CAD build for the part. Positions are in the model's coordinates, mm. Face numbers are marked on the shaded views. A direction names the side the tool comes from. Give positions to 0.01 mm unless a question says otherwise; leave off trailing zeros. Order: outer loops, then holes, each group sorted by start corner. A loop starts at its lowest first (then second) coordinate and runs counter-clockwise, first axis right, second up.
Item 1: Flat gauge pins, fed straight in: P1, Ø9.5, axis at y = 8, z = 0.5, coming from the -X side; P2, Ø7, axis at x = -80, z = -13, coming from the +Y side. Where does each tip first touch, or does it go through?
Item 2: Band-saw the part on C-C on x = -37.5. Give the cut face in (y, z).
Item 3: Which spindle directions (+Z, -Z, +X, -X, +Y, -Y) get a long thin tool onto all of the face, cutting with end or side? Do the marked faces 1, 2 and 3. Say none if no direction does.
Item 4: Band-saw the part on D-D on y = 3.75. Count the separate pieces of the cut face and the enclosed holes in it, plus the area to 3 significant figures.
Item 5: Band-saw the part on B-B on x = -80. Give the cut face in (y, z), plus the area to 3 significant figures.
Item 6: Two-plate mould, pull along X, no slides. Class the marked faces 4, 5, 6 and 7: released by +X, released by -X, zero draft, split by the parting line, or undercut.
Item 7: Band-saw the part on A-A on x = -11.25. Give the cut face in (y, z), plus the area to 3 significant figures.
Item 8: Wall check: L1, parallel to Z at x = -80, y = 6; L2, parallel to Z at x = -74.5, y = 5; L3, parallel to X at y = 8.5, z = 1. Give the ranges that are in metal, low to high.
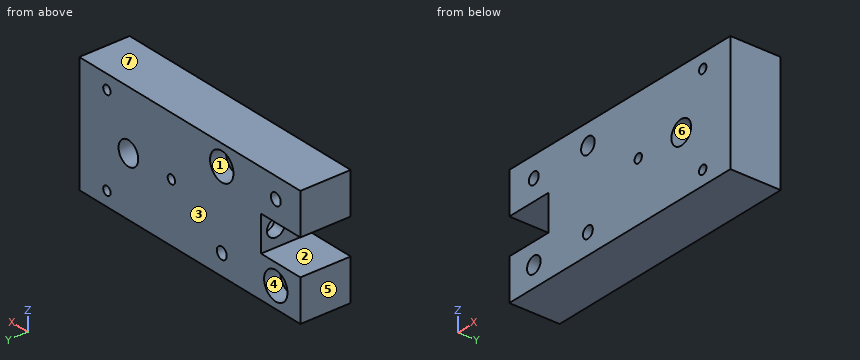
```python
from build123d import *

# Parameters (mm, degrees)
EXTRUDE_1_DEPTH        = 17
SKETCH_4_R             = 2.75
SKETCH_4_R_2           = 2
SKETCH_4_R_3           = 4
SKETCH_4_R_4           = 1.5
CUT_EXTRUDE_2_DEPTH    = 18
SKETCH_5_R             = 4.75
CUT_EXTRUDE_3_DEPTH    = 5.4
HOLE_WIZARD_M4_1_D     = 6
HOLE_WIZARD_M4_1_DEPTH = 4
HOLE_WIZARD_M4_1_TIP   = 1.802581857


with BuildPart() as part:
    # 스케치1 → 보스-돌출1 (new body)
    with BuildSketch(Plane(origin=(0, 0, 0), x_dir=(1, 0, 0), z_dir=(0, 1, 0))):
        Polygon((-90, -6), (-90, -20), (0, -20), (0, 20), (-90, 20), (-90, 6), (-74, 6), (-74, -6), align=None)
    extrude(amount=EXTRUDE_1_DEPTH)

    # 스케치4 → 컷-돌출2 (cut, through all)
    with BuildSketch(Plane.XZ):
        with Locations((-80, -13)):
            Circle(SKETCH_4_R)
        with Locations((-80, 13)):
            Circle(SKETCH_4_R_2)
        with Locations((-58, 13)):
            Circle(SKETCH_4_R)
        with Locations((-58, -13)):
            Circle(SKETCH_4_R_2)
        with Locations((-20, 0)):
            Circle(SKETCH_4_R_3)
        with Locations((-11.25, 15.155444566)):
            Circle(SKETCH_4_R_4)
        with Locations((-11.25, -15.155444566)):
            Circle(SKETCH_4_R_4)
        with Locations((-37.5, 0)):
            Circle(SKETCH_4_R_4)
    extrude(amount=-CUT_EXTRUDE_2_DEPTH, mode=Mode.SUBTRACT)

    # 스케치5 → 컷-돌출3 (cut)
    with BuildSketch(Plane(origin=(0, 17, 0), x_dir=(1, 0, 0), z_dir=(0, 1, 0))):
        with Locations((-80, 13)):
            Circle(SKETCH_5_R)
        with Locations((-58, -13)):
            Circle(SKETCH_5_R)
    extrude(amount=-CUT_EXTRUDE_3_DEPTH, mode=Mode.SUBTRACT)

    # M4 여유 구멍1
    with Locations(Plane.ZY.offset(74)):
        with Locations((0, 12)):
            Hole(HOLE_WIZARD_M4_1_D / 2, depth=HOLE_WIZARD_M4_1_DEPTH)
            with Locations((0, 0, -(HOLE_WIZARD_M4_1_DEPTH + HOLE_WIZARD_M4_1_TIP / 2))):  # 118° drill point
                Cone(0, HOLE_WIZARD_M4_1_D / 2, HOLE_WIZARD_M4_1_TIP, mode=Mode.SUBTRACT)


solid = part.part
```
The answers:
1. P1: stops at x = -74
1. P2: stops at y = 11.6
2. outline: (0, -20) - (17, -20) - (17, -1.5) - (0, -1.5) - close; (0, 1.5) - (17, 1.5) - (17, 20) - (0, 20) - close
3. face 1: +Y
3. face 2: -X, +Y, -Y
3. face 3: +Z, -Z, +X, -X, +Y
4. separate pieces: 1
4. enclosed holes: 8
4. area: 3,260 mm2
5. outline: (0, -20) - (17, -20) - (17, -17.75) - (11.6, -17.75) - (11.6, -15.75) - (0, -15.75) - close; (0, -10.25) - (11.6, -10.25) - (11.6, -8.25) - (17, -8.25) - (17, -6) - (0, -6) - close; (0, 6) - (17, 6) - (17, 11) - (0, 11) - close; (0, 15) - (17, 15) - (17, 20) - (0, 20) - close
5. area: 293 mm2
6. face 4: undercut
6. face 5: released by -X
6. face 6: undercut
6. face 7: zero draft
7. outline: (0, -20) - (17, -20) - (17, -16.66) - (0, -16.66) - close; (0, -13.66) - (17, -13.66) - (17, 13.66) - (0, 13.66) - close; (0, 16.66) - (17, 16.66) - (17, 20) - (0, 20) - close
7. area: 578 mm2
8. L1: z = -20 to -15.75, -10.25 to -6, 6 to 11, 15 to 20
8. L2: z = -20 to -6, 6 to 20
8. L3: x = -74 to -38.62, -36.38 to -23.87, -16.13 to 0
